Build history of the part. All positions in model axes, mm. Face numbers are marked on the shaded views. Give positions to 0.01 mm unless a question says otherwise; leave off trailing zeros. Loops run counter-clockwise (first coordinate to the right, second up) from the corner with the lowest first, then second, coordinate; pieces in that order, holes last.
1) Band-saw the part on A-A on x = -44. List the corners of the cut face in (y, z), then the cut area to 3 significant figures.
2) Flat gauge pins, fed straight in: P1, Ø1.5, axis at x = -32.5, y = 1, coming from the +Z side; P2, Ø0.9, axis at x = 39, y = 1.5, coming from the -Z side; P3, Ø0.9, axis at y = 1.5, z = 34, coming from the +X side. Where does each tip first touch, or does it go through?
3) Band-saw the part on B-B on z = 4.5. List the corners of the cut face in (x, y), then the cut area to 3 significant figures.
4) Band-saw the part on C-C on x = -78.5. List the corners of the cut face in (y, z), then the cut area to 3 significant figures.
5) Wall check: line 1 (Z direction, x = -24, y = 1.8); line 2 (X direction, y = 0.8, z = 1); line 3 (X direction, y = 2.3, z = -68.5). Give the ranges that are in metal, low to high.
6) Two-plate mould, pull along Y, no slides. Class the marked faces 1 and 2: +Y half, -Y half, draft (parallel to the pull), parting line (faces both ways), or undercut.
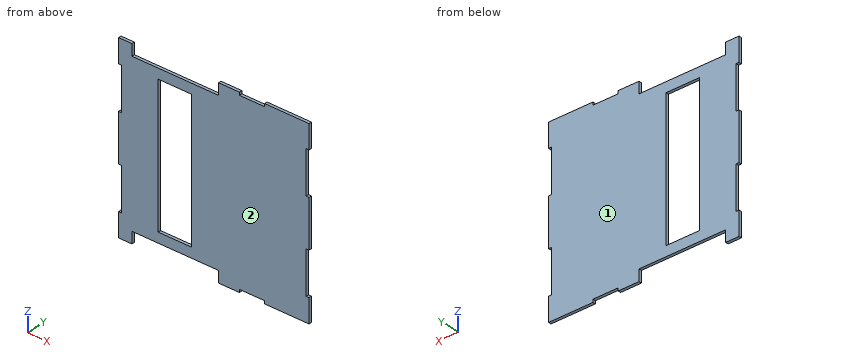
```python
from build123d import *

# Parameters (mm, degrees)
SKETCH1_W               = 200
SKETCH1_H               = 190
BOSS_EXTRUDE1_DEPTH     = 3
CUT_EXTRUDE2_DEPTH      = 138.963763358
CUT_EXTRUDE2_DEPTH_BACK = 3
SKETCH2_OUTSIDE_W       = 257.176
SKETCH2_OUTSIDE_H       = 247.176
SKETCH3_W               = 35
SKETCH3_H               = 145
CUT_EXTRUDE3_DEPTH      = 3
SKETCH4_W               = 90.968696296
SKETCH4_H               = 12
CUT_EXTRUDE4_DEPTH      = 3
SKETCH6_W               = 26.456316212
SKETCH6_H               = 3
CUT_EXTRUDE5_DEPTH      = 3


with BuildPart() as part:
    # Sketch1 → Boss-Extrude1 (new body)
    with BuildSketch(Plane(origin=(0, 0, 0), x_dir=(1, 0, 0), z_dir=(0, 1, 0))):
        Rectangle(SKETCH1_W, SKETCH1_H)
    extrude(amount=BOSS_EXTRUDE1_DEPTH)

    # Sketch2 outside → Cut-Extrude2 (cut, two sides: drawn at the far end of the back side and taken through both)
    with BuildSketch(Plane(origin=(0, 3, 0), x_dir=(1, 0, 0), z_dir=(0, 1, 0)).offset(-CUT_EXTRUDE2_DEPTH_BACK)):
        Rectangle(SKETCH2_OUTSIDE_W, SKETCH2_OUTSIDE_H)
        Polygon((-100, -95), (-100, -70), (-97, -70), (-97, -25), (-100, -25), (-100, 25), (-97, 25), (-97, 70), (-100, 70), (-100, 95), (100, 95), (100, 70), (97, 70), (97, 25), (100, 25), (100, -25), (97, -25), (97, -70), (100, -70), (100, -95), align=None, mode=Mode.SUBTRACT)
    extrude(amount=CUT_EXTRUDE2_DEPTH + CUT_EXTRUDE2_DEPTH_BACK, mode=Mode.SUBTRACT)

    # Sketch3 → Cut-Extrude3 (cut)
    with BuildSketch(Plane(origin=(0, 3, 0), x_dir=(1, 0, 0), z_dir=(0, 1, 0))):
        with Locations((-40.873559806, 0)):
            Rectangle(SKETCH3_W, SKETCH3_H)
    extrude(amount=-CUT_EXTRUDE3_DEPTH, mode=Mode.SUBTRACT)

    # Sketch4 → Cut-Extrude4 (cut)
    with BuildSketch(Plane(origin=(0, 3, 0), x_dir=(1, 0, 0), z_dir=(0, 1, 0))):
        with Locations((-40.484348148, 89)):
            Rectangle(SKETCH4_W, SKETCH4_H)
        with Locations((-40.484348148, -89)):
            Rectangle(SKETCH4_W, SKETCH4_H)
    extrude(amount=-CUT_EXTRUDE4_DEPTH, mode=Mode.SUBTRACT)

    # Sketch6 → Cut-Extrude5 (cut)
    with BuildSketch(Plane.XY.offset(95)):
        with Locations((40.079944256, 1.5)):
            Rectangle(SKETCH6_W, SKETCH6_H)
        Polygon((28.711773307, -23.399830076), (27.78877695, -20.614939543), (57.834413552, -10.656913259), (58.805651465, -13.58735957), align=None)
    cut_extrude5 = extrude(amount=-CUT_EXTRUDE5_DEPTH, mode=Mode.SUBTRACT)

    # Mirror1: Cut-Extrude5 across plane
    add(cut_extrude5.mirror(Plane.XY), mode=Mode.SUBTRACT)


solid = part.part
```
Findings below:
1. outline: (0, -83) - (3, -83) - (3, -72.5) - (0, -72.5) - close; (0, 72.5) - (3, 72.5) - (3, 83) - (0, 83) - close
1. area: 63.0 mm2
2. P1: stops at z = 83
2. P2: stops at z = -92
2. P3: stops at x = 97
3. outline: (-100, 0) - (-58.37, 0) - (-58.37, 3) - (-100, 3) - close; (-23.37, 0) - (100, 0) - (100, 3) - (-23.37, 3) - close
3. area: 495 mm2
4. outline: (0, -83) - (3, -83) - (3, 83) - (0, 83) - close
4. area: 498 mm2
5. line 1: z = -83 to -72.5, 72.5 to 83
5. line 2: x = -100 to -58.37, -23.37 to 100
5. line 3: x = -97 to -58.37, -23.37 to 97
6. face 1: +Y half
6. face 2: -Y half
